Can you work these out from the model? Positions are in its coordinate system, mm. A direction names the side the tool comes from. Round coordinates to 2 decimals unless told otherwise and drop trailing zeros. Write each loop counter-clockwise with the first axis right and the second up, starting at its lowest first coordinate (ties: lowest second). Pieces come first, ordered by that corner, then holes. Notation, with made-up numbers: M -2.5,-23 L 5.5,-23 A15 ccw 5.5,-6 Z; hole C 11,82.25 d2. An arc over 180 degrees is marked long. Answer as a JSON object with one key per item and string values. Group by question number.
1) Suppose I cut it at D-D, the plane x = 31. Write out the boundary of the cut face in (y, z).
2) I'm going to push flat-ended pins straight in: pin 1 Ø0.5 at (y, z) = (2.5, 0.5) entering from +X; pin 2 Ø4 at (x, y) = (21, 7) entering from -Z; pin 3 Ø0.5 at (x, z) = (35.5, 0.5) entering from -Y. Where does each tip first touch, or does it pass through?
3) Suppose I cut it at B-B, the plane y = 6.5. State how many separate pieces and enclosed holes the cut face has, and give its area (3 significant figures).
4) Please list where these lines run through material, in increasing order: L1, parallel to Y at x = 22, z = 0.3; L2, parallel to X at y = 6.25, z = 0.9; L3, parallel to X at y = 7.25, z = 0.5. Write a range as [from, to].
5) On a 3-axis mill with a long thin cutter (end or side, diameter ignored), from which of +Z, -Z, +X, -X, +Y, -Y can I reach the whole of each face in a straight line? I mean faces 1 (the flat face through (0, 7.9, 0.5)), 2 (the flat face through (21.4, 15, 0.5)), 3 (the flat face through (21.1, 1, 0.5)). Say none if no direction works.
6) Suppose I cut it at A-A, the plane x = 37.5. Write out the boundary of the cut face in (y, z), and give its area (3 significant figures).
from build123d import *

# Parameters (mm, degrees)
SKETCH001_R      = 2.5
EXTRUDE001_DEPTH = 1
SKETCH035_R      = 2
SKETCH036_R      = 1
SKETCH040_R      = 2
SKETCH038_R      = 1
SKETCH041_R      = 2
SKETCH039_R      = 1
SKETCH037_R      = 2
SKETCH034_R      = 1
SKETCH017_R      = 2
SKETCH016_R      = 1
SKETCH011_R      = 2
SKETCH010_R      = 1
SKETCH025_R      = 2
SKETCH024_R      = 1
SKETCH019_R      = 2
SKETCH018_R      = 1
SKETCH015_R      = 2
SKETCH014_R      = 1
SKETCH023_R      = 2
SKETCH022_R      = 1
SKETCH021_R      = 2
SKETCH020_R      = 1
SKETCH013_R      = 2
SKETCH012_R      = 1
SKETCH029_R      = 2
SKETCH028_R      = 1
SKETCH031_R      = 2
SKETCH030_R      = 1
SKETCH033_R      = 2
SKETCH032_R      = 1
SKETCH027_R      = 2
SKETCH026_R      = 1
SKETCH005_R      = 2
SKETCH004_R      = 1
SKETCH009_R      = 2
SKETCH008_R      = 1
SKETCH002_R      = 2
SKETCH003_R      = 1
SKETCH007_R      = 2
SKETCH006_R      = 1
EXTRUDE_DEPTH    = 1


with BuildPart() as extrude001:
    # Sketch001 → Extrude001 (new body)
    with BuildSketch(Plane(origin=(-2, 0, 0), x_dir=(1, 0, 0), z_dir=(0, 0, 1))):
        with Locations((39.5, 8)):
            Circle(SKETCH001_R)
    extrude(amount=EXTRUDE001_DEPTH)


with BuildPart() as loft017:
    # Sketch035 → Loft017 section 0
    with BuildSketch(Plane.XY.offset(1)):
        with Locations((2, 2)):
            Circle(SKETCH035_R)
    # Sketch036 → Loft017 section 1
    with BuildSketch(Plane.XY):
        with Locations((2, 2)):
            Circle(SKETCH036_R)
    loft()


with BuildPart() as loft017_1:
    # Loft017 placement: moved
    add(loft017.part.moved(Location((14, 11, 0))))


with BuildPart() as loft018:
    # Sketch040 → Loft018 section 0
    with BuildSketch(Plane.XY.offset(1)):
        with Locations((2, 2)):
            Circle(SKETCH040_R)
    # Sketch038 → Loft018 section 1
    with BuildSketch(Plane.XY):
        with Locations((2, 2)):
            Circle(SKETCH038_R)
    loft()


with BuildPart() as loft018_1:
    # Loft018 placement: moved
    add(loft018.part.moved(Location((20, 11, 0))))


with BuildPart() as loft019:
    # Sketch041 → Loft019 section 0
    with BuildSketch(Plane.XY.offset(1)):
        with Locations((2, 2)):
            Circle(SKETCH041_R)
    # Sketch039 → Loft019 section 1
    with BuildSketch(Plane.XY):
        with Locations((2, 2)):
            Circle(SKETCH039_R)
    loft()


with BuildPart() as loft019_1:
    # Loft019 placement: moved
    add(loft019.part.moved(Location((26, 11, 0))))


with BuildPart() as fusion001:
    # Sketch037 → Loft016 section 0
    with BuildSketch(Plane.XY.offset(1)):
        with Locations((2, 2)):
            Circle(SKETCH037_R)
    # Sketch034 → Loft016 section 1
    with BuildSketch(Plane.XY):
        with Locations((2, 2)):
            Circle(SKETCH034_R)
    loft()


with BuildPart() as fusion001_1:
    # Loft016 placement: moved
    add(fusion001.part.moved(Location((8, 11, 0))))

    # Fusion001: union Loft017, Loft018, Loft019
    add(loft017_1.part)
    add(loft018_1.part)
    add(loft019_1.part)


with BuildPart() as loft007:
    # Sketch017 → Loft007 section 0
    with BuildSketch(Plane.XY.offset(1)):
        with Locations((2, 2)):
            Circle(SKETCH017_R)
    # Sketch016 → Loft007 section 1
    with BuildSketch(Plane.XY):
        with Locations((2, 2)):
            Circle(SKETCH016_R)
    loft()


with BuildPart() as loft007_1:
    # Loft007 placement: moved
    add(loft007.part.moved(Location((11, 4, 0))))


with BuildPart() as loft004:
    # Sketch011 → Loft004 section 0
    with BuildSketch(Plane.XY.offset(1)):
        with Locations((2, 2)):
            Circle(SKETCH011_R)
    # Sketch010 → Loft004 section 1
    with BuildSketch(Plane.XY):
        with Locations((2, 2)):
            Circle(SKETCH010_R)
    loft()


with BuildPart() as loft004_1:
    # Loft004 placement: moved
    add(loft004.part.moved(Location((5, 4, 0))))


with BuildPart() as loft011:
    # Sketch025 → Loft011 section 0
    with BuildSketch(Plane.XY.offset(1)):
        with Locations((2, 2)):
            Circle(SKETCH025_R)
    # Sketch024 → Loft011 section 1
    with BuildSketch(Plane.XY):
        with Locations((2, 2)):
            Circle(SKETCH024_R)
    loft()


with BuildPart() as loft011_1:
    # Loft011 placement: moved
    add(loft011.part.moved(Location((23, 4, 0))))


with BuildPart() as fusion003:
    # Sketch019 → Loft008 section 0
    with BuildSketch(Plane.XY.offset(1)):
        with Locations((2, 2)):
            Circle(SKETCH019_R)
    # Sketch018 → Loft008 section 1
    with BuildSketch(Plane.XY):
        with Locations((2, 2)):
            Circle(SKETCH018_R)
    loft()


with BuildPart() as fusion003_1:
    # Loft008 placement: moved
    add(fusion003.part.moved(Location((17, 4, 0))))

    # Fusion003: union Loft007, Loft004, Loft011
    add(loft007_1.part)
    add(loft004_1.part)
    add(loft011_1.part)


with BuildPart() as fusion003_2:
    # Fusion003 placement: moved
    add(fusion003_1.part.moved(Location((0.001, -0.001, 0))))


with BuildPart() as loft006:
    # Sketch015 → Loft006 section 0
    with BuildSketch(Plane.XY.offset(1)):
        with Locations((2, 2)):
            Circle(SKETCH015_R)
    # Sketch014 → Loft006 section 1
    with BuildSketch(Plane.XY):
        with Locations((2, 2)):
            Circle(SKETCH014_R)
    loft()


with BuildPart() as loft006_1:
    # Loft006 placement: moved
    add(loft006.part.moved(Location((11, 8, 0))))


with BuildPart() as loft010:
    # Sketch023 → Loft010 section 0
    with BuildSketch(Plane.XY.offset(1)):
        with Locations((2, 2)):
            Circle(SKETCH023_R)
    # Sketch022 → Loft010 section 1
    with BuildSketch(Plane.XY):
        with Locations((2, 2)):
            Circle(SKETCH022_R)
    loft()


with BuildPart() as loft010_1:
    # Loft010 placement: moved
    add(loft010.part.moved(Location((23, 8, 0))))


with BuildPart() as loft009:
    # Sketch021 → Loft009 section 0
    with BuildSketch(Plane.XY.offset(1)):
        with Locations((2, 2)):
            Circle(SKETCH021_R)
    # Sketch020 → Loft009 section 1
    with BuildSketch(Plane.XY):
        with Locations((2, 2)):
            Circle(SKETCH020_R)
    loft()


with BuildPart() as loft009_1:
    # Loft009 placement: moved
    add(loft009.part.moved(Location((17, 8, 0))))


with BuildPart() as fusion007:
    # Sketch013 → Loft005 section 0
    with BuildSketch(Plane.XY.offset(1)):
        with Locations((2, 2)):
            Circle(SKETCH013_R)
    # Sketch012 → Loft005 section 1
    with BuildSketch(Plane.XY):
        with Locations((2, 2)):
            Circle(SKETCH012_R)
    loft()


with BuildPart() as fusion007_1:
    # Loft005 placement: moved
    add(fusion007.part.moved(Location((5, 8, 0))))

    # Fusion002: union Loft006, Loft010, Loft009
    add(loft006_1.part)
    add(loft010_1.part)
    add(loft009_1.part)


with BuildPart() as fusion007_2:
    # Fusion002 placement: moved
    add(fusion007_1.part.moved(Location((0.001, 0.001, 0))))

    # Fusion007: union Fusion003
    add(fusion003_2.part)


with BuildPart() as loft013:
    # Sketch029 → Loft013 section 0
    with BuildSketch(Plane.XY.offset(1)):
        with Locations((2, 2)):
            Circle(SKETCH029_R)
    # Sketch028 → Loft013 section 1
    with BuildSketch(Plane.XY):
        with Locations((2, 2)):
            Circle(SKETCH028_R)
    loft()


with BuildPart() as loft013_1:
    # Loft013 placement: moved
    add(loft013.part.moved(Location((14, 1, 0))))


with BuildPart() as loft014:
    # Sketch031 → Loft014 section 0
    with BuildSketch(Plane.XY.offset(1)):
        with Locations((2, 2)):
            Circle(SKETCH031_R)
    # Sketch030 → Loft014 section 1
    with BuildSketch(Plane.XY):
        with Locations((2, 2)):
            Circle(SKETCH030_R)
    loft()


with BuildPart() as loft014_1:
    # Loft014 placement: moved
    add(loft014.part.moved(Location((20, 1, 0))))


with BuildPart() as loft015:
    # Sketch033 → Loft015 section 0
    with BuildSketch(Plane.XY.offset(1)):
        with Locations((2, 2)):
            Circle(SKETCH033_R)
    # Sketch032 → Loft015 section 1
    with BuildSketch(Plane.XY):
        with Locations((2, 2)):
            Circle(SKETCH032_R)
    loft()


with BuildPart() as loft015_1:
    # Loft015 placement: moved
    add(loft015.part.moved(Location((26, 1, 0))))


with BuildPart() as fusion:
    # Sketch027 → Loft012 section 0
    with BuildSketch(Plane.XY.offset(1)):
        with Locations((2, 2)):
            Circle(SKETCH027_R)
    # Sketch026 → Loft012 section 1
    with BuildSketch(Plane.XY):
        with Locations((2, 2)):
            Circle(SKETCH026_R)
    loft()


with BuildPart() as fusion_1:
    # Loft012 placement: moved
    add(fusion.part.moved(Location((8, 1, 0))))

    # Fusion: union Loft013, Loft014, Loft015
    add(loft013_1.part)
    add(loft014_1.part)
    add(loft015_1.part)


with BuildPart() as loft001:
    # Sketch005 → Loft001 section 0
    with BuildSketch(Plane.XY.offset(1)):
        with Locations((2, 2)):
            Circle(SKETCH005_R)
    # Sketch004 → Loft001 section 1
    with BuildSketch(Plane.XY):
        with Locations((2, 2)):
            Circle(SKETCH004_R)
    loft()


with BuildPart() as loft001_1:
    # Loft001 placement: moved
    add(loft001.part.moved(Location((4, 0, 0))))


with BuildPart() as fusion004:
    # Sketch009 → Loft002 section 0
    with BuildSketch(Plane.XY.offset(1)):
        with Locations((2, 2)):
            Circle(SKETCH009_R)
    # Sketch008 → Loft002 section 1
    with BuildSketch(Plane.XY):
        with Locations((2, 2)):
            Circle(SKETCH008_R)
    loft()


with BuildPart() as fusion004_1:
    # Loft002 placement: moved
    add(fusion004.part.moved(Location((4, 12, 0))))

    # Fusion004: union Loft001
    add(loft001_1.part)


with BuildPart() as loft_body:
    # Sketch002 → Loft section 0
    with BuildSketch(Plane.XY.offset(1)):
        with Locations((2, 2)):
            Circle(SKETCH002_R)
    # Sketch003 → Loft section 1
    with BuildSketch(Plane.XY):
        with Locations((2, 2)):
            Circle(SKETCH003_R)
    loft()


with BuildPart() as fusion008:
    # Sketch007 → Loft003 section 0
    with BuildSketch(Plane.XY.offset(1)):
        with Locations((2, 2)):
            Circle(SKETCH007_R)
    # Sketch006 → Loft003 section 1
    with BuildSketch(Plane.XY):
        with Locations((2, 2)):
            Circle(SKETCH006_R)
    loft()


with BuildPart() as fusion008_1:
    # Loft003 placement: moved
    add(fusion008.part.moved(Location((0, 12, 0))))

    # Fusion005: union Loft body
    add(loft_body.part)


with BuildPart() as fusion008_2:
    # Fusion005 placement: moved
    add(fusion008_1.part.moved(Location((-0.001, 0, 0))))

    # Fusion006: union Fusion004
    add(fusion004_1.part)

    # Fusion008: union Fusion001, Fusion007, Fusion
    add(fusion001_1.part)
    add(fusion007_2.part)
    add(fusion_1.part)


with BuildPart() as obj1:
    # Sketch → Extrude (new body)
    with BuildSketch(Plane.XY):
        with BuildLine():
            Line((0, 0.999999), (0, 15))
            ThreePointArc((1, 16), (0.292893, 15.707107), (0, 15))
            Line((1, 16), (7.5, 16))
            ThreePointArc((8, 15.5), (7.853553, 15.853554), (7.5, 16))
            ThreePointArc((8, 15.5), (8.146447, 15.146447), (8.5, 15))
            Line((34, 15), (8.5, 15))
            ThreePointArc((35, 14), (34.707107, 14.707107), (34, 15))
            Line((35, 14), (35, 13))
            Line((35, 13), (37.000002, 13))
            ThreePointArc((37.000002, 3), (42, 8), (37.000002, 13))
            Line((37.000002, 3), (35, 3))
            Line((35, 2), (35, 3))
            ThreePointArc((34, 1), (34.707107, 1.292893), (35, 2))
            Line((8.5, 1), (34, 1))
            ThreePointArc((8.5, 1), (8.146447, 0.853553), (8, 0.5))
            ThreePointArc((7.5, 0), (7.853553, 0.146446), (8, 0.5))
            Line((7.5, 0), (1, 0))
            ThreePointArc((0, 0.999999), (0.292893, 0.292893), (1, 0))
        make_face()
    extrude(amount=EXTRUDE_DEPTH)

    # Cut: cut Fusion008
    add(fusion008_2.part, mode=Mode.SUBTRACT)

    # Cut001: cut Extrude001
    add(extrude001.part, mode=Mode.SUBTRACT)


solid = obj1.part
Results:
{
 "1": {"outline": "M 1,0 L 15,0 L 15,1 L 1,1 Z"},
 "2": {"pin 1": "x = 35", "pin 2": "z = 0", "pin 3": "y = 3"},
 "3": {"separate pieces": "6", "enclosed holes": "0", "area": "26.5 mm^2"},
 "4": {"L1": "[1, 1.7], [4.3, 11.7], [14.3, 15]", "L2": "[0, 5.12], [8.88, 11.12], [14.88, 17.12], [20.88, 23.12], [26.88, 35.71], [39.29, 41.68]", "L3": "[0, 6.17], [7.83, 12.17], [13.83, 18.17], [19.83, 24.17], [25.83, 35.12], [39.88, 41.94]"},
 "5": {"face 1": "+Z, -Z, -X, +Y, -Y", "face 2": "+Z, -Z, +X, +Y", "face 3": "+Z, -Z, +X, -Y"},
 "6": {"outline": "M 3.03,0 L 5.5,0 L 5.5,1 L 3.03,1 Z; M 10.5,0 L 12.97,0 L 12.97,1 L 10.5,1 Z", "area": "4.95 mm^2"}
}
